```python
from build123d import *

# Parameters (mm, degrees)
SKETCH1_W               = 30
SKETCH1_H               = 20
BOSS_EXTRUDE1_DEPTH     = 4
SKETCH2_W               = 30
SKETCH2_H               = 4
BOSS_EXTRUDE2_DEPTH     = 15
CUT_EXTRUDE1_DEPTH      = 2.5
SKETCH4_R               = 1
CUT_EXTRUDE2_DEPTH      = 19.5
CUT_EXTRUDE2_DEPTH_BACK = 2.5
CUT_EXTRUDE3_DEPTH      = 16
CUT_EXTRUDE3_DEPTH_BACK = 2.5
SKETCH6_R               = 1
CUT_EXTRUDE4_DEPTH      = 18.5
CUT_EXTRUDE4_DEPTH_BACK = 2.5


with BuildPart() as part:
    # Sketch1 → Boss-Extrude1 (new body)
    with BuildSketch(Plane(origin=(0, 0, 0), x_dir=(1, 0, 0), z_dir=(0, 1, 0))):
        Rectangle(SKETCH1_W, SKETCH1_H)
    extrude(amount=BOSS_EXTRUDE1_DEPTH)

    # Sketch2 → Boss-Extrude2 (add)
    with BuildSketch(Plane(origin=(0, 4, 0), x_dir=(1, 0, 0), z_dir=(0, 1, 0))):
        with Locations((0, 8)):
            Rectangle(SKETCH2_W, SKETCH2_H)
    extrude(amount=BOSS_EXTRUDE2_DEPTH)

    # Sketch3 → Cut-Extrude1 (cut)
    with BuildSketch(Plane.XY.offset(-6)):
        Polygon((-8.874166975, 12.771236672), (-7.74833395, 14.721236672), (-8.874166975, 16.671236672), (-11.125833025, 16.671236672), (-12.25166605, 14.721236672), (-11.125833025, 12.771236672), align=None)
        Polygon((1.140266782, 12.743045001), (2.280533563, 14.718045001), (1.140266782, 16.693045001), (-1.140266782, 16.693045001), (-2.280533563, 14.718045001), (-1.140266782, 12.743045001), align=None)
        Polygon((12.028231439, 12.721236672), (13.182931977, 14.721236672), (12.028231439, 16.721236672), (9.718830362, 16.721236672), (8.564129823, 14.721236672), (9.718830362, 12.721236672), align=None)
        Polygon((-4.580088939, 6.006448413), (-3.410954644, 8.031448413), (-4.580088939, 10.056448413), (-6.91835753, 10.056448413), (-8.087491825, 8.031448413), (-6.91835753, 6.006448413), align=None)
        Polygon((6.807808173, 5.981448413), (7.991376224, 8.031448413), (6.807808173, 10.081448413), (4.440672069, 10.081448413), (3.257104017, 8.031448413), (4.440672069, 5.981448413), align=None)
    extrude(amount=-CUT_EXTRUDE1_DEPTH, mode=Mode.SUBTRACT)

    # Sketch4 → Cut-Extrude2 (cut, two sides)
    with BuildSketch(Plane.XY.offset(-8.5)) as cut_extrude2_sk:
        with Locations((-10, 14.721236672)):
            Circle(SKETCH4_R)
        with Locations((0, 14.718045001)):
            Circle(SKETCH4_R)
        with Locations((10.8735309, 14.721236672)):
            Circle(SKETCH4_R)
        with Locations((5.624240121, 8.031448413)):
            Circle(SKETCH4_R)
        with Locations((-5.749223235, 8.031448413)):
            Circle(SKETCH4_R)
    extrude(amount=CUT_EXTRUDE2_DEPTH, mode=Mode.SUBTRACT)
    extrude(cut_extrude2_sk.sketch, amount=-CUT_EXTRUDE2_DEPTH_BACK, mode=Mode.SUBTRACT)

    # Sketch5 → Cut-Extrude3 (cut, two sides)
    with BuildSketch(Plane(origin=(0, 4, 0), x_dir=(1, 0, 0), z_dir=(0, 1, 0))) as cut_extrude3_sk:
        Polygon((-10.310121887, -0.481448413), (-9.184288862, 1.468551587), (-10.310121887, 3.418551587), (-12.561787937, 3.418551587), (-13.687620962, 1.468551587), (-12.561787937, -0.481448413), align=None)
        Polygon((-0.64074259, -0.506448413), (0.499524192, 1.468551587), (-0.64074259, 3.443551587), (-2.921276153, 3.443551587), (-4.061542935, 1.468551587), (-2.921276153, -0.506448413), align=None)
        Polygon((9.091128264, -0.531448413), (10.245828803, 1.468551587), (9.091128264, 3.468551587), (6.781727188, 3.468551587), (5.627026649, 1.468551587), (6.781727188, -0.531448413), align=None)
        Polygon((-5.798674299, -7.368028115), (-4.629540004, -5.343028115), (-5.798674299, -3.318028115), (-8.136942889, -3.318028115), (-9.306077184, -5.343028115), (-8.136942889, -7.368028115), align=None)
        Polygon((4.745586795, -7.205553444), (5.929154847, -5.155553444), (4.745586795, -3.105553444), (2.378450691, -3.105553444), (1.194882639, -5.155553444), (2.378450691, -7.205553444), align=None)
    extrude(amount=CUT_EXTRUDE3_DEPTH, mode=Mode.SUBTRACT)
    extrude(cut_extrude3_sk.sketch, amount=-CUT_EXTRUDE3_DEPTH_BACK, mode=Mode.SUBTRACT)

    # Sketch6 → Cut-Extrude4 (cut, two sides)
    with BuildSketch(Plane(origin=(0, 1.5, 0), x_dir=(1, 0, 0), z_dir=(0, 1, 0))) as cut_extrude4_sk:
        with Locations((-11.435954912, 1.468551587)):
            Circle(SKETCH6_R)
        with Locations((-1.781009372, 1.468551587)):
            Circle(SKETCH6_R)
        with Locations((7.936427726, 1.468551587)):
            Circle(SKETCH6_R)
        with Locations((3.562018743, -5.155553444)):
            Circle(SKETCH6_R)
        with Locations((-6.967808594, -5.343028115)):
            Circle(SKETCH6_R)
    extrude(amount=CUT_EXTRUDE4_DEPTH, mode=Mode.SUBTRACT)
    extrude(cut_extrude4_sk.sketch, amount=-CUT_EXTRUDE4_DEPTH_BACK, mode=Mode.SUBTRACT)


solid = part.part
```
Model file for the job. Use its own axes, mm. A direction names the side the tool comes from. Coordinates: 2 decimals unless noted, no trailing zeros. Order: outer loops, then holes, each group sorted by start corner. A loop starts at its lowest first (then second) coordinate and runs counter-clockwise, first axis right, second up. Notation, with made-up numbers: (80.5, 9) -> (103.5, 9) arc R6 ccw to (103.5, 18) -> close; hole circle Ø10 at (63, -7). An arc over 180 degrees is marked (long way). Answer as a JSON object with one key per item and string values. Group by question number.
1) Cut at D-D, the plane y = 18.25. Write the cut outline in (x, z).
2) Pull direction Z, two halves, no side cores. Call faces 1 (the face through (0, 16, -8.5)), 2 (the face through (11, 12.721, -7)), 3 (the face through (5.346, 2.768, 4.145)): +Z half, -Z half, draft (parallel to the pull), parting line (faces both ways), or undercut.
3) Cut at C-C, the plane x = -7.25. Write the cut outline in (y, z).
4) Drill centre lines: L1, parallel to Y at x = -5.25, z = -6.25; L2, parallel to X at y = 14.5, z = -6.75; L3, parallel to Y at x = 0, z = -9.05. Where is each one in solid material? Low to high.
5) Cut at A-A, the plane x = 0. Write the cut outline in (y, z).
6) Flat gauge pins, fed straight in: pin 1 (12 mm diameter, centred on x = -3, z = 1, fed in from +Y); pin 2 (1.2 mm diameter, centred on x = 3.56, z = 5.16, fed in from -Y); pin 3 (1.2 mm diameter, centred on x = 4.5, z = 4.5, fed in from +Y); pin 4 (4.5 mm diameter, centred on x = -1, y = 15.5, fed in from +Z). Where does each tip first touch, or does it go through?
7) Cut at B-B, the plane y = 2.5. Count the separate pieces of the cut face and the enclosed holes in it, then the cut area to 3 significant figures.
8) Which spindle directions (+Z, -Z, +X, -X, +Y, -Y) get a long thin tool onto all of the face, cutting with end or side? Do faces 4 (the face through (4, 3, 7.206)), 5 (the face through (-0.217, 13.742, -9.24)), 6 (the face through (1.702, 13.717, -7.232)). Say none if no direction does.
Check values:
{
 "1": {"outline": "(-15, -10) -> (15, -10) -> (15, -6) -> (-15, -6) -> close"},
 "2": {"face 1": "+Z half", "face 2": "draft", "face 3": "undercut"},
 "3": {"outline": "(0, -10) -> (19, -10) -> (19, -6) -> (9.48, -6) -> (9.48, -8.5) -> (6.58, -8.5) -> (6.58, -6) -> (4, -6) -> (4, 3.32) -> (1.5, 3.32) -> (1.5, 4.38) -> (0, 4.38) -> close; (0, 6.3) -> (1.5, 6.3) -> (1.5, 7.37) -> (4, 7.37) -> (4, 10) -> (0, 10) -> close"},
 "4": {"L1": "y = 0 to 6.01, 10.06 to 19", "L2": "x = -15 to -12.12, -7.88 to -2.15, 2.15 to 8.69, 13.06 to 15", "L3": "y = 0 to 13.72, 15.72 to 19"},
 "5": {"outline": "(0, -10) -> (13.72, -10) -> (13.72, -8.5) -> (12.74, -8.5) -> (12.74, -6) -> (4, -6) -> (4, -2.33) -> (1.5, -2.33) -> (1.5, -0.6) -> (4, -0.6) -> (4, 10) -> (0, 10) -> close; (15.72, -10) -> (19, -10) -> (19, -6) -> (16.69, -6) -> (16.69, -8.5) -> (15.72, -8.5) -> close"},
 "6": {"pin 1": "stops at y = 4", "pin 2": "passes through", "pin 3": "stops at y = 1.5", "pin 4": "stops at z = -6"},
 "7": {"separate pieces": "1", "enclosed holes": "5", "area": "531 mm²"},
 "8": {"face 4": "+Y", "face 5": "+Z, -Z", "face 6": "+Z"}
}
